Part model, mm, in its own coordinate system. A direction names the side the tool comes from. Round coordinates to 2 decimals unless told otherwise and drop trailing zeros. Loops run counter-clockwise (first coordinate to the right, second up) from the corner with the lowest first, then second, coordinate; pieces in that order, holes last. Notation, with made-up numbers: M 29.25,20 L 70.25,20 A27 ccw 70.25,40 Z; hole C 13,29.5 d6. An arc over 180 degrees is marked long. Put each result on its own line as item: value. Start each with the question number.
1) Which spindle directions (+Z, -Z, +X, -X, +Y, -Y) get a long thin tool onto all of the face, cutting with end or side? Do faces 1 (the flat face through (-42.621, 2, -35)), 2 (the flat face through (-1, 2, -39.1)), 3 (the flat face through (-37.033, 2, 35)). Say none if no direction does.
2) Pull direction X, two halves, no side cores. Call faces 4 (the flat face through (40, 2, -31.48)), 5 (the flat face through (-67.691, 2, -1)), 6 (the flat face through (55, 2, -39.1)), 7 (the cylindrical face through (-1.68, 2.254, 9.987)): +X half, -X half, draft (parallel to the pull), parting line (faces both ways), or undercut.
3) Slice it at D-D on z = 11.7. Give the cut face in (x, y).
4) Slice it at C-C on y = 3.1. Give the cut face in (x, z) (1 decimal).
5) Drop flat-ended pins along their axis: pin 1 Ø3 at (x, z) = (-1.905, 11.7) entering from -Y; pin 2 Ø2 at (x, y) = (40, 3) entering from -Z. Give the stop position or say it passes through.
6) Probe line 1 along X through (y, z) = (1.8, 11.7); line 2 along X through (y, z) = (3.75, -28); line 3 along Z through (x, y) = (-58.42, 3.1). List the from-to ranges inside material, lowest first.
7) Slice it at B-B on x = -58.42. Give the cut face in (y, z).
8) Slice it at A-A on z = -27.67. Give the cut face in (x, y), then the cut area to 3 significant figures.
```python
from build123d import *

# Parameters (mm, degrees)
SKETCH1_W              = 135.382
SKETCH1_H              = 62.96
SKETCH1_W_2            = 25.0698
SKETCH1_H_2            = 7.62
SKETCH1_W_3            = 74.0664
BOSS_EXTRUDE1_DEPTH    = 4.572
F_10_32_TAPPED_HOLE1_D = 4.0386
F_8_32_TAPPED_HOLE1_D  = 3.4544


with BuildPart() as part:
    # Sketch1 → Boss-Extrude1 (new body)
    with BuildSketch(Plane(origin=(0, 0, 0), x_dir=(1, 0, 0), z_dir=(0, 1, 0))):
        Rectangle(SKETCH1_W, SKETCH1_H)
        with Locations((55.1561, 35.29)):
            Rectangle(SKETCH1_W_2, SKETCH1_H_2)
        with Locations((0, 35.29)):
            Rectangle(SKETCH1_W_3, SKETCH1_H_2)
        with Locations((-55.1561, 35.29)):
            Rectangle(SKETCH1_W_2, SKETCH1_H_2)
        with Locations((-55.1561, -35.29)):
            Rectangle(SKETCH1_W_2, SKETCH1_H_2)
        with Locations((0, -35.29)):
            Rectangle(SKETCH1_W_3, SKETCH1_H_2)
        with Locations((55.1561, -35.29)):
            Rectangle(SKETCH1_W_2, SKETCH1_H_2)
    extrude(amount=BOSS_EXTRUDE1_DEPTH)

    # #10-32 Tapped Hole1 (through all)
    with Locations(Plane(origin=(0, 4.572, 0), x_dir=(1, 0, 0), z_dir=(0, 1, 0))):
        with Locations((-58.42, 27.67), (32.0675, 27.67)):
            Hole(F_10_32_TAPPED_HOLE1_D / 2)

    # #8-32 Tapped Hole1 (through all)
    with Locations(Plane(origin=(0, 4.572, 0), x_dir=(1, 0, 0), z_dir=(0, 1, 0))):
        with Locations((-29.845, -11.7), (-1.905, -11.7)):
            Hole(F_8_32_TAPPED_HOLE1_D / 2)


solid = part.part
```
Recorded:
1. face 1: -Z, +Y, -Y
1. face 2: -Z, +X, -X, +Y, -Y
1. face 3: +Z, +Y, -Y
2. face 4: undercut
2. face 5: -X half
2. face 6: draft
2. face 7: undercut
3. outline: M -67.69,0 L -31.57,0 L -31.57,4.57 L -67.69,4.57 Z; M -28.12,0 L -3.63,0 L -3.63,4.57 L -28.12,4.57 Z; M -0.18,0 L 67.69,0 L 67.69,4.57 L -0.18,4.57 Z
4. outline: M -67.7,-39.1 L -42.6,-39.1 L -42.6,-31.5 L -37,-31.5 L -37,-39.1 L 37,-39.1 L 37,-31.5 L 42.6,-31.5 L 42.6,-39.1 L 67.7,-39.1 L 67.7,39.1 L 42.6,39.1 L 42.6,31.5 L 37,31.5 L 37,39.1 L -37,39.1 L -37,31.5 L -42.6,31.5 L -42.6,39.1 L -67.7,39.1 Z; hole C -58.4,-27.7 d4; hole C -29.8,11.7 d3.5; hole C -1.9,11.7 d3.5; hole C 32.1,-27.7 d4
5. pin 1: passes through
5. pin 2: stops at z = -31.48
6. line 1: x = -67.69 to -31.57, -28.12 to -3.63, -0.18 to 67.69
6. line 2: x = -67.69 to -60.41, -56.43 to 30.08, 34.06 to 67.69
6. line 3: z = -39.1 to -29.69, -25.65 to 39.1
7. outline: M 0,-39.1 L 4.57,-39.1 L 4.57,-29.69 L 0,-29.69 Z; M 0,-25.65 L 4.57,-25.65 L 4.57,39.1 L 0,39.1 Z
8. outline: M -67.69,0 L -60.44,0 L -60.44,4.57 L -67.69,4.57 Z; M -56.4,0 L 30.05,0 L 30.05,4.57 L -56.4,4.57 Z; M 34.09,0 L 67.69,0 L 67.69,4.57 L 34.09,4.57 Z
8. area: 582 mm2
